Source: CAD feature listing. Evaluate the final solid. Frame: model axes, mm. A direction names the side the tool comes from. Give positions to 0.01 mm unless a question says otherwise; leave off trailing zeros. Write each loop counter-clockwise with the first axis right and the second up, starting at its lowest first coordinate (ties: lowest second). Pieces come first, ordered by that corner, then holes. Notation, with made-up numbers: (15.25, 46) - (44.25, 46) arc R21 ccw to (44.25, 50) - close; hole circle Ø1 at (-4, -25.75). An arc over 180 degrees is marked (long way). One line per question, with ' | ' between items. Start each with the question number.
(1) Section A-A, the plane y = 5.5. Return loops of the section in (x, z), plus the area to 3 significant figures.
(2) Ray query, line 1 (Y direction, x = -0.5, z = 5.45); line 2 (Y direction, x = -0.5, z = 1.15); line 3 (X direction, y = -5.5, z = 4.5). Return the intervals inside material, ascending. Write a range as [from, to].
(3) Pin query (flat end, axial travel): pin 1 (2.5 mm diameter, centred on x = 0.5, y = 6.5, fed in from -Z). Return the tip coordinate at first contact, or that it passes through.
(4) Section C-C, the plane z = 4. Return loops of the section in (x, y).
(5) Section D-D, the plane z = 1. Return loops of the section in (x, y).
(6) Section B-B, the plane x = -0.5. State how many separate pieces and enclosed holes the cut face has, plus the area to 3 significant figures.
(7) Draft query along Y for faces 3 (the flat face through (0, 9.5, 4)), 4 (the flat face through (-3, 0, 5)), 5 (the cylindrical face through (-0.56, -6.97, 5.39)). Return one class per face: +Y half, -Y half, draft (parallel to the pull), parting line (faces both ways), or undercut.
(8) Access query for faces 1 (the flat face through (0, -9.5, 4)), 2 (the cylindrical face through (2.277, -5.597, 1.467)). Directions: +Z, -Z, +X, -X, +Y, -Y. A direction counts if a zero-diameter tool reaches every point of the face in a straight line with its end or side. Return the directions, or none.
```python
from build123d import *

# Parameters (mm, degrees)
SKETCH_1_W                = 6
SKETCH_1_H                = 19
EXTRUDE_1_DEPTH           = 8
HOLE_WIZARD_41_AT_2_COUNT = 2
HOLE_WIZARD_41_AT_2_PITCH = 11
CHAMFER_1_SIZE            = 0.449397949


with BuildPart() as part:
    # Эскиз1 → Бобышка-Вытянуть1 (new body)
    with BuildSketch(Plane.XY):
        Rectangle(SKETCH_1_W, SKETCH_1_H)
    extrude(amount=EXTRUDE_1_DEPTH)

    # Эскиз2 → Цековка для  винта с внутренним шестигранником #41 (revolve, cut)
    with BuildSketch(Plane(origin=(-0.5, 5.5, 0), x_dir=(0, 1, 0), z_dir=(1, 0, 0))):
        Polygon((0, 0), (0, 8), (1.6002, 8), (1.4732, 7.873), (1.4732, 2.9718), (1.6002, 2.8448), (2.77876, 2.8448), (2.77876, 0.127), (2.90576, 0), align=None)
    hole_wizard_41 = revolve(axis=Axis((-0.5, 5.5, -6.35), (0, 0, 1)), mode=Mode.SUBTRACT)

    # Цековка для  винта с внутренним шестигранником #41 at 2: Цековка для  винта с внутренним шестигранником #41 ×2
    with Locations(*[(0, -i * HOLE_WIZARD_41_AT_2_PITCH, 0) for i in range(1, HOLE_WIZARD_41_AT_2_COUNT)]):
        add(hole_wizard_41, mode=Mode.SUBTRACT)

    # Фаска1
    # the kernel refuses this chamfer: 0.5, 0.449397949 mm, written as the material it takes off along each edge
    with BuildSketch(Plane(origin=(-3, -4.286943061, 2.8448), x_dir=(0.5198491944846588, 0.8542580494169495, 0), z_dir=(0, 0, -1)), Plane(origin=(-3, 6.713056939, 2.8448), x_dir=(0.5198491944846584, 0.8542580494169496, 0), z_dir=(0, 0, -1))) as chamfer_1_piece_1:
        with BuildLine():
            Line((0.526718663, 0), (CHAMFER_1_SIZE * 0.854258048776, -CHAMFER_1_SIZE * 0.519849194094))
            Line((CHAMFER_1_SIZE * 0.854258048776, -CHAMFER_1_SIZE * 0.519849194094), (0, 0))
            ThreePointArc((0, 0), (0.268614935, -0.012503234), (0.526718663, 0))
        make_face()
    extrude(amount=4.061353185, mode=Mode.SUBTRACT)
    with BuildSketch(Plane(origin=(-3, -6.713056939, 2.8448), x_dir=(0.519849194484659, -0.8542580494169493, 0), z_dir=(0, 0, -1)), Plane(origin=(-3, 4.286943061, 2.8448), x_dir=(0.519849194484659, -0.8542580494169493, 0), z_dir=(0, 0, -1))) as chamfer_1_piece_2:
        with BuildLine():
            Line((0.526718663, 0), (CHAMFER_1_SIZE * 0.854258048776, CHAMFER_1_SIZE * 0.519849194094))
            Line((CHAMFER_1_SIZE * 0.854258048776, CHAMFER_1_SIZE * 0.519849194094), (0, 0))
            ThreePointArc((0, 0), (0.268614935, 0.012503234), (0.526718663, 0))
        make_face()
    extrude(amount=4.061353185, mode=Mode.SUBTRACT)


solid = part.part
```
Check sheet entries:
1) outline: (-3, 2.84) - (-2.1, 2.84) - (-1.97, 2.97) - (-1.97, 7.87) - (-2.1, 8) - (-3, 8) - close; (0.97, 2.97) - (1.1, 2.84) - (2.28, 2.84) - (2.28, 0.13) - (2.41, 0) - (3, 0) - (3, 8) - (1.1, 8) - (0.97, 7.87) - close | area: 17.8 mm²
2) line 1: [-9.5, -6.97], [-4.03, 4.03], [6.97, 9.5] | line 2: [-9.5, -8.28], [-2.72, 2.72], [8.28, 9.5] | line 3: [-3, -1.97], [0.97, 3]
3) pin 1: z = 2.84
4) outline: (-3, -9.5) - (3, -9.5) - (3, 9.5) - (-3, 9.5) - close; hole circle Ø2.95 at (-0.5, -5.5); hole circle Ø2.95 at (-0.5, 5.5)
5) outline: (-3, -9.5) - (3, -9.5) - (3, 9.5) - (-3, 9.5) - (-3, 7.16) - (-2.73, 7.16) arc R2.78 cw (long way) to (-2.73, 3.84) - (-3, 3.84) - (-3, -3.84) - (-2.73, -3.84) arc R2.78 cw (long way) to (-2.73, -7.16) - (-3, -7.16) - close
6) separate pieces: 3 | enclosed holes: 0 | area: 89.9 mm²
7) face 3: +Y half | face 4: draft | face 5: undercut
8) face 1: +Z, -Z, +X, -X, -Y | face 2: -Z
